Design review of the part shown in the three views and the two pictorial views. Dimensions are in mm from the part's minimum x, y and z. A direction names the side the tool comes from. Round coordinates to 2 decimals unless told otherwise and drop trailing zeros. Loops run counter-clockwise (first coordinate to the right, second up) from the corner with the lowest first, then second, coordinate; pieces in that order, holes last.
1) Wall thickness on L1, parallel to Y at x = 45, z = 6; L2, parallel to X at y = 7.5, z = 13.5; L3, parallel to Y at x = 5.5, z = 6.25: over which ranges is each line inside the solid? List them lowest first.
2) Take a section at D-D (y = 41). State the section outline as (x, z) points.
3) Tool access review of the marked faces 5, 6 and 7: name each direction out of +Z, -Z, +X, -X, +Y, -Y from which nothing blocks a thin tool from reaching the whole face with its end or side.
4) Insertion check: pin 1 (10 mm diameter, centred on x = 37, z = 4.5, fed in from -Y); pin 2 (2 mm diameter, centred on x = 45, y = 45, fed in from +Z); pin 3 (4 mm diameter, centred on x = 28.5, y = 7.5, fed in from +Z). Each pin has a flat end and moves straight along its axis. Give the tip position at first contact, or say it passes through.
5) Take a section at B-B (y = 5). State the section outline as (x, z) points.
6) Take a section at C-C (x = 5). State the section outline as (y, z) points.
7) Mouldability with a two-part tool opening along X and no side actions: class the marked faces 1, 2, 3 and 4 as pulls with the +X half, pulls with the -X half, needs draft (parallel to the pull), parting line crosses it, or undercut.
8) Take a section at A-A (z = 20). State the section outline as (x, y) points.
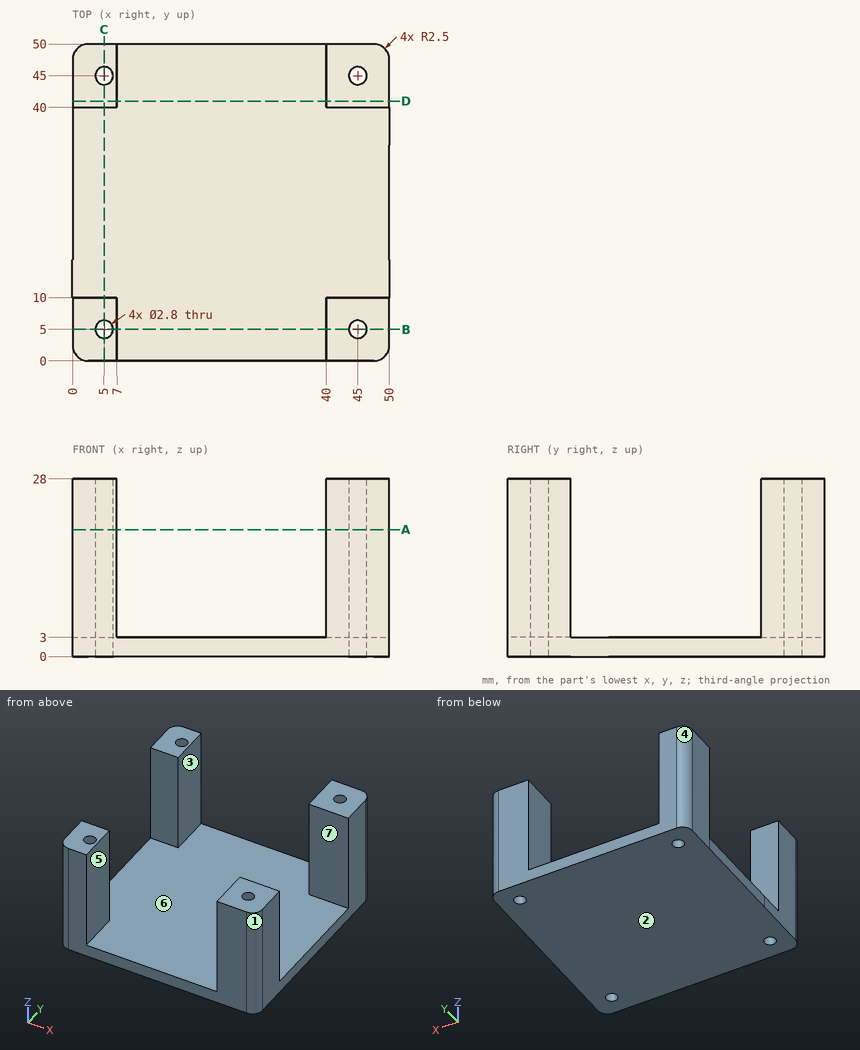
Response:
1. L1: y = 0 to 3.6, 6.4 to 10, 40 to 43.6, 46.4 to 50
1. L2: x = 0 to 7, 40 to 50
1. L3: y = 0 to 3.69, 6.31 to 10, 40 to 43.69, 46.31 to 50
2. outline: (0, 0) - (50, 0) - (50, 28) - (40, 28) - (40, 3) - (7, 3) - (7, 28) - (0, 28) - close
3. face 5: +Z, +Y, -Y
3. face 6: +Z
3. face 7: +Z, +X, -X
4. pin 1: stops at y = 0
4. pin 2: passes through
4. pin 3: stops at z = 3
5. outline: (0, 0) - (3.6, 0) - (3.6, 28) - (0, 28) - close; (6.4, 0) - (43.6, 0) - (43.6, 28) - (40, 28) - (40, 3) - (7, 3) - (7, 28) - (6.4, 28) - close; (46.4, 0) - (50, 0) - (50, 28) - (46.4, 28) - close
6. outline: (0, 0) - (3.6, 0) - (3.6, 28) - (0, 28) - close; (6.4, 0) - (43.6, 0) - (43.6, 28) - (40, 28) - (40, 3) - (10, 3) - (10, 28) - (6.4, 28) - close; (46.4, 0) - (50, 0) - (50, 28) - (46.4, 28) - close
7. face 1: pulls with the +X half
7. face 2: needs draft
7. face 3: undercut
7. face 4: pulls with the -X half
8. outline: (0, 2.5) arc R2.5 ccw to (2.5, 0) - (7, 0) - (7, 10) - (0, 10) - close; (0, 40) - (7, 40) - (7, 50) - (2.5, 50) arc R2.5 ccw to (0, 47.5) - close; (40, 0) - (47.5, 0) arc R2.5 ccw to (50, 2.5) - (50, 10) - (40, 10) - close; (40, 40) - (50, 40) - (50, 47.5) arc R2.5 ccw to (47.5, 50) - (40, 50) - close; hole circle Ø2.8 at (5, 5); hole circle Ø2.8 at (5, 45); hole circle Ø2.8 at (45, 5); hole circle Ø2.8 at (45, 45)
